Part print with two shaded views. Sizes in mm from the minimum x, y, z corner. Round coordinates to 2 decimals unless told otherwise and drop trailing zeros. Loops run counter-clockwise (first coordinate to the right, second up) from the corner with the lowest first, then second, coordinate; pieces in that order, holes last. Notation, with made-up numbers: (62, 24.25) - (82, 24.25) arc R11 ccw to (82, 36.25) - close; hole circle Ø5 at (73, 56.5). An arc over 180 degrees is marked (long way). Use a Markdown table: item, result.
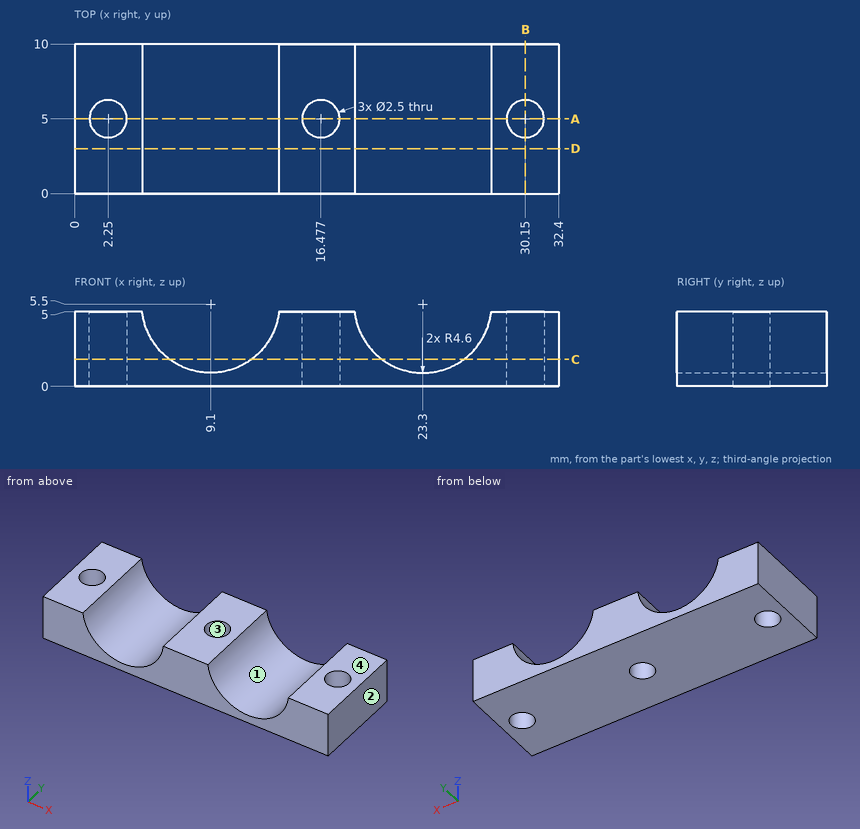
Q1. Cut at A-A, the plane y = 5. List the corners of the cut face in (x, z).
Results found:
| item | result |
|---|---|
| outline | (0, 0) - (1, 0) - (1, 5) - (0, 5) - close; (3.5, 0) - (15.23, 0) - (15.23, 5) - (13.67, 5) arc R4.6 cw to (4.53, 5) - (3.5, 5) - close; (17.73, 0) - (28.9, 0) - (28.9, 5) - (27.87, 5) arc R4.6 cw to (18.73, 5) - (17.73, 5) - close; (31.4, 0) - (32.4, 0) - (32.4, 5) - (31.4, 5) - close |
Q2. Probe line 1 (Y direction, x = 2.25, z = 3.35); line 2 (X direction, y = 8, z = 4.6); line 3 (X direction, y = 9.25, z = 3.3). List the from-to ranges inside material, lowest first.
Results found:
| item | result |
|---|---|
| line 1 | y = 0 to 3.75, 6.25 to 10 |
| line 2 | x = 0 to 4.59, 13.61 to 18.79, 27.81 to 32.4 |
| line 3 | x = 0 to 5.06, 13.14 to 19.26, 27.34 to 32.4 |
Q3. Cut at C-C, the plane z = 1.8. List the corners of the cut face in (x, y).
Results found:
| item | result |
|---|---|
| outline | (0, 0) - (6.37, 0) - (6.37, 10) - (0, 10) - close; (11.83, 0) - (20.57, 0) - (20.57, 10) - (11.83, 10) - close; (26.03, 0) - (32.4, 0) - (32.4, 10) - (26.03, 10) - close; hole circle Ø2.5 at (2.25, 5); hole circle Ø2.5 at (16.48, 5); hole circle Ø2.5 at (30.15, 5) |
Q4. Cut at B-B, the plane x = 30.15. List the corners of the cut face in (y, z), plus the area to 3 significant figures.
Results found:
| item | result |
|---|---|
| outline | (0, 0) - (3.75, 0) - (3.75, 5) - (0, 5) - close; (6.25, 0) - (10, 0) - (10, 5) - (6.25, 5) - close |
| area | 37.5 mm2 |
Q5. Drop flat-ended pins along their axis: pin 1 (2 mm diameter, centred on x = 12, y = 4, fed in from +Z); pin 2 (1 mm diameter, centred on x = 8.5, y = 3, fed in from +Z). Give the stop position or say it passes through.
Results found:
| item | result |
|---|---|
| pin 1 | stops at z = 3.06 |
| pin 2 | stops at z = 1.03 |
Q6. Pull direction X, two halves, no side cores. Call the marked faces 1, 2, 3 and 4: pulls with the +X half, pulls with the -X half, needs draft (parallel to the pull), parting line crosses it, or undercut.
Results found:
| item | result |
|---|---|
| face 1 | undercut |
| face 2 | pulls with the +X half |
| face 3 | undercut |
| face 4 | needs draft |
Q7. Cut at D-D, the plane y = 3. List the corners of the cut face in (x, z).
Results found:
| item | result |
|---|---|
| outline | (0, 0) - (32.4, 0) - (32.4, 5) - (27.87, 5) arc R4.6 cw to (18.73, 5) - (13.67, 5) arc R4.6 cw to (4.53, 5) - (0, 5) - close |
